Geometry: final body of the model. Coordinates: model frame, mm. Face numbers are marked on the shaded views. A direction names the side the tool comes from. Give positions to 0.01 mm unless a question says otherwise; leave off trailing zeros. Write each loop counter-clockwise with the first axis right and the second up, starting at its lowest first coordinate (ties: lowest second). Pieces come first, ordered by that corner, then holes. Notation, with made-up numbers: M 42.25,23 L 95.25,23 A25 cw 95.25,47 Z; hole C -27,15 d10. An arc over 180 degrees is marked long. Use one line per item in the form item = value. Start each with the question number.
Item 1: Section query A-A on y = 32. Return loops of the section in (x, z).
Item 2: Access query for the marked faces 1, 2, 3 and 4. Directions: +Z, -Z, +X, -X, +Y, -Y. A direction counts if a zero-diameter tool reaches every point of the face in a straight line with its end or side. Return the directions, or none.
Item 3: Pull-direction query (X, two-part tool) for the marked faces 5, 6 and 7; classes: released by +X, released by -X, zero draft, split by the parting line, or undercut.
Item 4: Material intervals for line 1 along Z through (x, y) = (10, 33.5); line 2 along X through (y, z) = (33, 9.25); line 3 along X through (y, z) = (8, 6.5), sorted ascending. Write a range as from..to.
Item 5: Contact query for flat-ended pins moving along their axis: P1, Ø3, axis at x = 43.5, z = 5.5, coming from the -Y side; P2, Ø5, axis at x = 22.5, z = 2.5, coming from the -Y side; P3, Ø3, axis at y = 23.5, z = 8, coming from the +X side; P4, Ø3, axis at y = 19, z = 3, coming from the -X side. Output: stop coordinate, or through.
Item 6: Section query C-C on z = 5. Return loops of the section in (x, y).
Item 7: Section query B-B on x = 10. Return loops of the section in (y, z).
Item 8: Section query D-D on y = 25. Return loops of the section in (x, z), then the cut area to 3 significant figures.
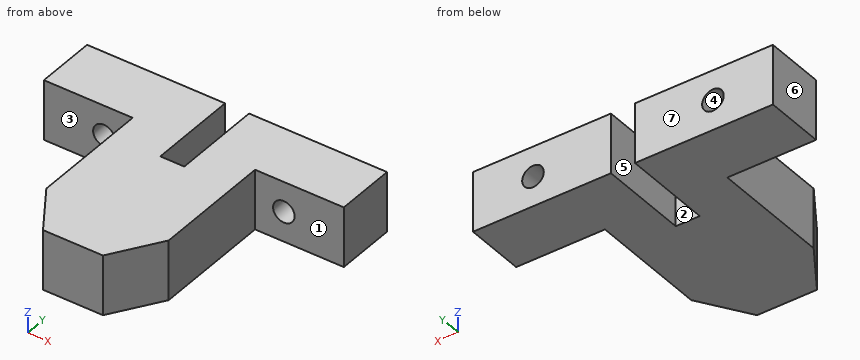
from build123d import *

# Parameters (mm, degrees)
SKETCH1_W           = 50
SKETCH1_H           = 38
BOSS_EXTRUDE1_DEPTH = 10
SKETCH2_R           = 1.8
CUT_EXTRUDE1_DEPTH  = 64.592452382
SKETCH3_W           = 4
SKETCH3_H           = 15
CUT_EXTRUDE2_DEPTH  = 10
CUT_EXTRUDE3_DEPTH  = 64.592452382


with BuildPart() as part:
    # Sketch1 → Boss-Extrude1 (new body)
    with BuildSketch(Plane.XY):
        with Locations((25, 19)):
            Rectangle(SKETCH1_W, SKETCH1_H)
    extrude(amount=BOSS_EXTRUDE1_DEPTH)

    # Sketch2 → Cut-Extrude1 (cut, through all)
    with BuildSketch(Plane(origin=(0, 38, 0), x_dir=(1, 0, 0), z_dir=(0, 1, 0))):
        with Locations(Location((10, -5, 0), (0, 0, 180))):
            Circle(SKETCH2_R)
        with Locations(Location((40, -5, 0), (0, 0, 180))):
            Circle(SKETCH2_R)
    extrude(amount=-CUT_EXTRUDE1_DEPTH, mode=Mode.SUBTRACT)

    # Sketch3 → Cut-Extrude2 (cut)
    with BuildSketch(Plane.XY.offset(10)):
        with Locations((25, 30.5)):
            Rectangle(SKETCH3_W, SKETCH3_H)
    extrude(amount=-CUT_EXTRUDE2_DEPTH, mode=Mode.SUBTRACT)

    # Sketch4 → Cut-Extrude3 (cut, through all)
    with BuildSketch(Plane.XY.offset(10)):
        Polygon((0, 28), (14.8, 28), (14.8, 8), (20, 0), (30, 0), (35.2, 8), (35.2, 28), (50, 28), (50, -1), (0, -1), align=None)
    extrude(amount=-CUT_EXTRUDE3_DEPTH, mode=Mode.SUBTRACT)


solid = part.part
Answer sheet:
q1.outline = M 0,0 L 23,0 L 23,10 L 0,10 Z; M 27,0 L 50,0 L 50,10 L 27,10 Z; hole C 10,5 d3.6; hole C 40,5 d3.6
q2.face_1 = +Z, -Z, +X, -Y
q2.face_2 = +Z, -Z, +Y
q2.face_3 = +Z, -Z, -X, -Y
q2.face_4 = +Y, -Y
q3.face_5 = undercut
q3.face_6 = released by -X
q3.face_7 = zero draft
q4.line_1 = 0..3.2, 6.8..10
q4.line_2 = 0..23, 27..50
q4.line_3 = 14.8..35.2
q5.P1 = 28
q5.P2 = 0
q5.P3 = 35.2
q5.P4 = 14.8
q6.outline = M 0,28 L 8.2,28 L 8.2,38 L 0,38 Z; M 11.8,28 L 14.8,28 L 14.8,8 L 20,0 L 30,0 L 35.2,8 L 35.2,28 L 38.2,28 L 38.2,38 L 27,38 L 27,23 L 23,23 L 23,38 L 11.8,38 Z; M 41.8,28 L 50,28 L 50,38 L 41.8,38 Z
q7.outline = M 28,0 L 38,0 L 38,3.2 L 28,3.2 Z; M 28,6.8 L 38,6.8 L 38,10 L 28,10 Z
q8.outline = M 14.8,0 L 23,0 L 23,10 L 14.8,10 Z; M 27,0 L 35.2,0 L 35.2,10 L 27,10 Z
q8.area = 164 mm2
